Source: three-view drawing plus pictorial views. Frame: mm from the lowest corner of the part. A direction names the side the tool comes from. Give positions to 0.01 mm unless a question says otherwise; leave off trailing zeros. Loops run counter-clockwise (first coordinate to the right, second up) from the corner with the lowest first, then second, coordinate; pieces in that order, holes last. Notation, with made-up numbers: (66, 54) - (87, 54) arc R26 cw to (87, 81) - close; hole circle Ø2 at (9, -29.75). An arc over 180 degrees is marked (long way). Answer as a JSON object with one key per item and string values. Group by question number.
(1) Material intervals for L1, parallel to Y at x = 37, z = 10; L2, parallel to Z at x = 53.5, y = 37.5; L3, parallel to X at y = 31, z = 14, sorted ascending.
(2) Section query B-B (x = 31.5). Return loops of the section in (y, z).
(3) Access query for the marked faces 1, 2 and 3. Directions: +Z, -Z, +X, -X, +Y, -Y. A direction counts if a zero-diameter tool reaches every point of the face in a straight line with its end or side. Return the directions, or none.
(4) Section query A-A (y = 20). Return loops of the section in (x, z), plus the area to 3 significant figures.
(5) Section query D-D (x = 21). Return loops of the section in (y, z), plus the area to 3 significant figures.
(6) Pin query (flat end, axial travel): P1, Ø10, axis at y = 26, z = 7.5, coming from the -X side; P2, Ø6, axis at y = 19.5, z = 7.5, coming from the +X side; P3, Ø6, axis at x = 22, y = 5, coming from the -Z side. Return the tip coordinate at first contact, or that it passes through.
(7) Section query C-C (y = 8.5). Return loops of the section in (x, z), plus the area to 3 significant figures.
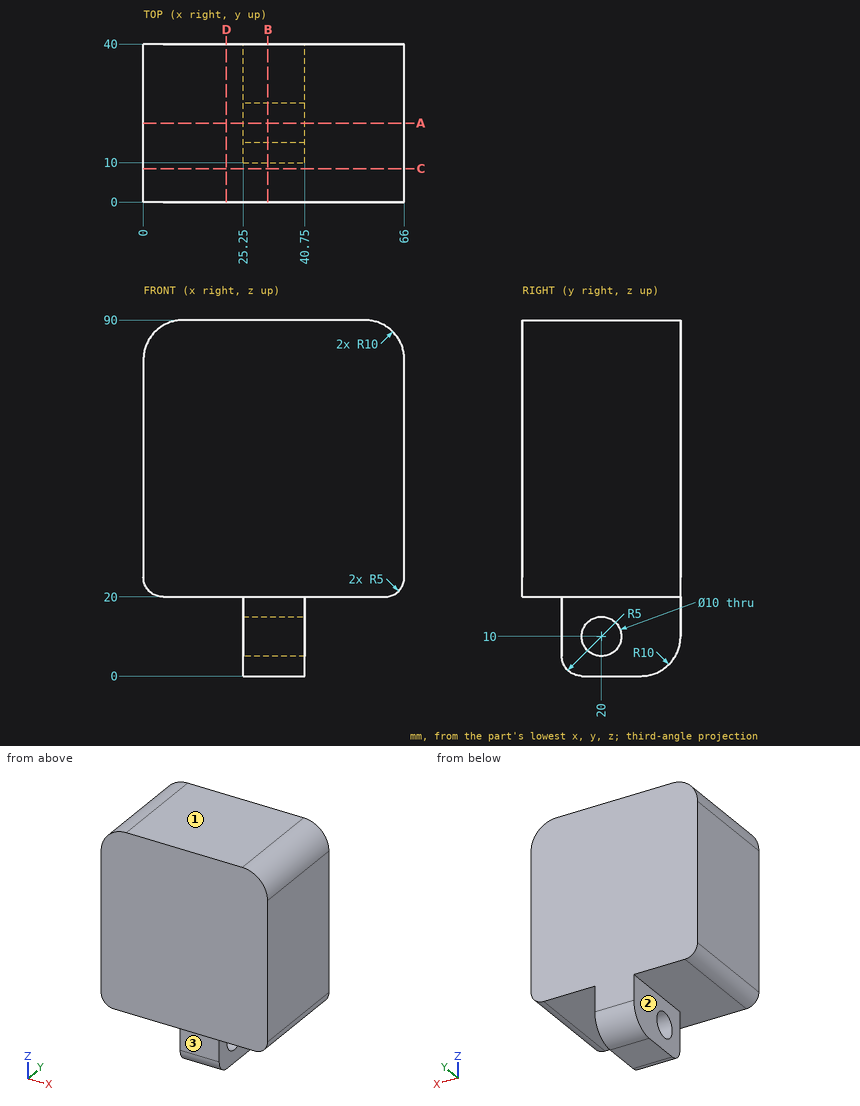
Recorded:
{
 "1": {"L1": "y = 10 to 15, 25 to 40", "L2": "z = 20 to 90", "L3": "x = 25.25 to 40.75"},
 "2": {"outline": "(0, 20) - (10, 20) - (10, 5) arc R5 ccw to (15, 0) - (30, 0) arc R10 ccw to (40, 10) - (40, 90) - (0, 90) - close; hole circle Ø10 at (20, 10)"},
 "3": {"face 1": "+Z, +X, -X, +Y, -Y", "face 2": "-Z, -X, +Y, -Y", "face 3": "-Z, +X, -X, -Y"},
 "4": {"outline": "(0, 25) arc R5 ccw to (5, 20) - (25.25, 20) - (25.25, 15) - (40.75, 15) - (40.75, 20) - (61, 20) arc R5 ccw to (66, 25) - (66, 80) arc R10 ccw to (56, 90) - (10, 90) arc R10 ccw to (0, 80) - close; (25.25, 0) - (40.75, 0) - (40.75, 5) - (25.25, 5) - close", "area": "4,720 mm^2"},
 "5": {"outline": "(0, 20) - (40, 20) - (40, 90) - (0, 90) - close", "area": "2,800 mm^2"},
 "6": {"P1": "stops at x = 25.25", "P2": "stops at x = 40.75", "P3": "stops at z = 20"},
 "7": {"outline": "(0, 25) arc R5 ccw to (5, 20) - (61, 20) arc R5 ccw to (66, 25) - (66, 80) arc R10 ccw to (56, 90) - (10, 90) arc R10 ccw to (0, 80) - close", "area": "4,570 mm^2"}
}
